```python
from build123d import *

# Parameters (mm, degrees)
F1_DEPTH = 60


with BuildPart() as f1:
    # F0 (on Top) → F1 (new body)
    with BuildSketch(Plane.XY):
        Polygon((-37.77854, 46.809994), (-32.797566, 46.374216), (-32.349713, 51.493207), (-31.828278, 57.453238), (-36.618262, 57.872308), (-44.77854, 47.422415), align=None)
        Polygon((-32.349713, 51.493207), (-32.797566, 46.374216), (-27.816593, 45.938437), align=None)
        Polygon((-39.841805, 23.226772), (-34.822705, 23.226772), (-32.797566, 46.374216), (-37.77854, 46.809994), align=None)
        Polygon((-35.150788, 19.476772), (-52.150788, 19.476772), (-45.178328, -60.218804), (-37.104148, -60.218804), (-30.610643, 14.002301), (-30.189987, 18.810422), (-29.360409, 28.292544), (-27.816593, 45.938437), (-32.797566, 46.374216), (-34.822705, 23.226772), align=None)
        Polygon((-30.189987, 18.810422), (-30.610643, 14.002301), (-26.987346, 17.784758), (-26.421964, 24.247109), (-29.360409, 28.292544), align=None)
        with BuildLine():
            Line((-45.178328, -60.218804), (-52.150788, 19.476772))
            ThreePointArc((-52.150788, 19.476772), (-50.747534, -20.553253), (-45.178328, -60.218804))
        make_face()
    extrude(amount=F1_DEPTH)


solid = f1.part
```
Check sheet for the modelled part. Datum: model origin and axes. Units: mm. A direction names the side the tool comes from. Coordinates: 2 decimals unless noted, no trailing zeros. Order: outer loops, then holes, each group sorted by start corner. A loop starts at its lowest first (then second) coordinate and runs counter-clockwise, first axis right, second up. Notation, with made-up numbers: M -6,68 L 21,68 A5 ccw 21,74 Z; hole C 10,52 d4. An arc over 180 degrees is marked long. Write each question's results on one line, items separated by ' | '. Start each with the question number.
1. Material ranges on probe 1 along Y at (x, z) = (-42, 21); probe 2 along Y at (x, z) = (-42.75, 44); probe 3 along X at (y, z) = (-44, 6.5), recorded low to high.
2. Mould release check, pull along Y, two halves, no side actions. Record for faces 1 (the face through (-41, -60.219, 30)), 2 (the face through (-32.093, 54.432, 29.58)), 3 (the face through (-40.64, 52.72, 29.58)), 4 (the face through (-34.984, 21.378, 29.58)): +Y half, -Y half, draft (parallel to the pull), parting line (faces both ways), or undercut.
3. Cross-section at C-C on y = 8.5. Record the cut outline in (x, z).
4. Cross-section at D-D on x = -50.5. Record the cut outline in (y, z), and give its area (3 significant figures).
5. Go/stop test with flat-tipped pins: P1, Ø2, axis at x = -38.5, z = 50.5, coming from the +Y side; P2, Ø1.5, axis at x = -49, z = 35, coming from the +Y side. Record where each tip stops, or that it passes through.
6. Access from +Z, -Z, +X, -X, +Y, -Y to the whole of each face (thin tool, end or side, straight path). Record for faces 5 (the face through (-38.796, 35.183, 29.58)), 6 (the face through (-28.6, 37, 29.6)), 7 (the face through (-33.9, -23.6, 29.6)).
7. Cross-section at B-B on z = 42.5. Record the cut outline in (x, y).
8. Cross-section at A-A on x = -42.5. Record the cut outline in (y, z).
Checks:
1) probe 1: y = -60.22 to 19.48, 47.18 to 50.98 | probe 2: y = -60.22 to 19.48, 47.24 to 50.02 | probe 3: x = -47.97 to -35.69
2) face 1: -Y half | face 2: undercut | face 3: +Y half | face 4: undercut
3) outline: M -52.18,0 L -31.09,0 L -31.09,60 L -52.18,60 Z
4) outline: M -23.27,0 L 19.48,0 L 19.48,60 L -23.27,60 Z | area: 2,560 mm²
5) P1: stops at y = 56.74 | P2: stops at y = 19.48
6) face 5: +Z, -Z, -X | face 6: +Z, -Z, +X | face 7: +Z, -Z, +X, -Y
7) outline: M -52.15,19.48 A383.65 ccw -45.18,-60.22 L -37.1,-60.22 L -30.61,14 L -26.99,17.78 L -26.42,24.25 L -29.36,28.29 L -27.82,45.94 L -32.35,51.49 L -31.83,57.45 L -36.62,57.87 L -44.78,47.42 L -37.78,46.81 L -39.84,23.23 L -34.82,23.23 L -35.15,19.48 Z
8) outline: M -60.22,0 L 19.48,0 L 19.48,60 L -60.22,60 Z; M 47.22,0 L 50.34,0 L 50.34,60 L 47.22,60 Z
